Build history of the part. All positions in model axes, mm. Face numbers are marked on the shaded views. Give positions to 0.01 mm unless a question says otherwise; leave off trailing zeros. Order: outer loops, then holes, each group sorted by start corner. A loop starts at its lowest first (then second) coordinate and runs counter-clockwise, first axis right, second up. Notation, with made-up numbers: (31.5, -13) - (71.5, -13) arc R6 cw to (71.5, -8) - close; hole circle Ø4 at (-32.75, 6.25). An arc over 180 degrees is marked (long way). Use a Markdown table: item, result. Add a question column.
(1) Slice it at C-C (z = 1.05). Write the cut outline in (x, y).
(2) Slice it at B-B (y = 9.85). Write the cut outline in (x, z).
(3) Wall check: line 1 (X direction, y = 9.85, z = 1.5); line 2 (Y direction, x = 15, z = 0.85); line 3 (X direction, y = 9.25, z = 0.2). Give the ranges that are in metal, low to high.
(4) Mould opens along X. For the marked faces 1, 2, 3 and 4 say: +X half, -X half, draft (parallel to the pull), parting line (faces both ways), or undercut.
(5) Slice it at A-A (x = 5). Write the cut outline in (y, z), then the cut area to 3 significant figures.
(6) Flat gauge pin, fed straight in: pin 1 (3 mm diameter, centred on x = 5, y = 9.85, fed in from +Z). Where does the tip first touch, or does it go through?
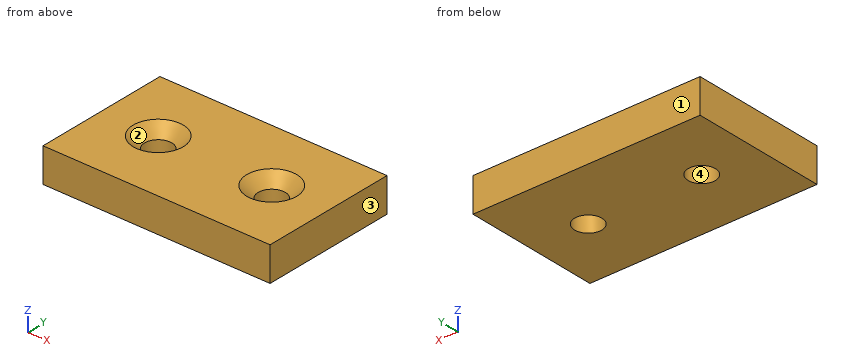
from build123d import *

# Parameters (mm, degrees)
SCHIZZO1_W                             = 20
SCHIZZO1_H                             = 19.7
ESTRUSIONE_ESTRUSIONE1_DEPTH           = 3
FORO_SVASATO_PER_VITE_M2_2_D           = 2.4
FORO_SVASATO_PER_VITE_M2_2_CSINK_D     = 4.4
FORO_SVASATO_PER_VITE_M2_2_CSINK_ANGLE = 90
SCHIZZO7_W                             = 20
SCHIZZO7_H                             = 3.85
TAGLIO_ESTRUSIONE1_DEPTH               = 10


with BuildPart() as part:
    # Schizzo1 → Estrusione-Estrusione1 (new body)
    with BuildSketch(Plane.XY):
        with Locations((10, 9.85)):
            Rectangle(SCHIZZO1_W, SCHIZZO1_H)
    extrude(amount=ESTRUSIONE_ESTRUSIONE1_DEPTH)

    # Foro svasato per Vite M2-2 (through all)
    with Locations(Plane.XY.offset(3)):
        with Locations((5, 9.85), (15, 9.85)):
            CounterSinkHole(FORO_SVASATO_PER_VITE_M2_2_D / 2, FORO_SVASATO_PER_VITE_M2_2_CSINK_D / 2, counter_sink_angle=FORO_SVASATO_PER_VITE_M2_2_CSINK_ANGLE)

    # Schizzo7 → Taglio-Estrusione1 (cut)
    with BuildSketch(Plane(origin=(0, 0, 0), x_dir=(-1, 0, 0), z_dir=(0, 0, -1))):
        with Locations((-10, 17.775)):
            Rectangle(SCHIZZO7_W, SCHIZZO7_H)
        with Locations((-10, 1.925)):
            Rectangle(SCHIZZO7_W, SCHIZZO7_H)
    extrude(amount=-TAGLIO_ESTRUSIONE1_DEPTH, mode=Mode.SUBTRACT)


solid = part.part
Solution:
| question | item | result |
|---|---|---|
| 1 | outline | (0, 3.85) - (20, 3.85) - (20, 15.85) - (0, 15.85) - close; hole circle Ø2.4 at (5, 9.85); hole circle Ø2.4 at (15, 9.85) |
| 2 | outline | (0, 0) - (3.8, 0) - (3.8, 2) - (2.8, 3) - (0, 3) - close; (6.2, 0) - (13.8, 0) - (13.8, 2) - (12.8, 3) - (7.2, 3) - (6.2, 2) - close; (16.2, 0) - (20, 0) - (20, 3) - (17.2, 3) - (16.2, 2) - close |
| 3 | line 1 | 0 to 3.8, 6.2 to 13.8, 16.2 to 20 |
| 3 | line 2 | 3.85 to 8.65, 11.05 to 15.85 |
| 3 | line 3 | 0 to 3.96, 6.04 to 13.96, 16.04 to 20 |
| 4 | face 1 | draft |
| 4 | face 2 | undercut |
| 4 | face 3 | +X half |
| 4 | face 4 | undercut |
| 5 | outline | (3.85, 0) - (8.65, 0) - (8.65, 2) - (7.65, 3) - (3.85, 3) - close; (11.05, 0) - (15.85, 0) - (15.85, 3) - (12.05, 3) - (11.05, 2) - close |
| 5 | area | 27.8 mm2 |
| 6 | pin 1 | z = 2.3 |
